```python
from build123d import *

# Parameters (mm, degrees)
SKETCH1_R                = 14.2875
BOSS_EXTRUDE2_DEPTH      = 3.175
BOSS_EXTRUDE2_DEPTH_BACK = 3.175


with BuildPart() as part:
    # Sketch1 → Boss-Extrude2 (new body, two sides)
    with BuildSketch(Plane(origin=(0, 0, 0), x_dir=(0, 0, -1), z_dir=(1, 0, 0))) as boss_extrude2_sk:
        with BuildLine():
            Line((10.594785966, 15.13092246), (203.963780766, 291.290466949))
            Line((203.963780766, 291.290466949), (110.334702104, 356.850253624))
            Line((110.334702104, 356.850253624), (-84.6362425, 78.402887714))
            ThreePointArc((-84.6362425, 78.402887714), (-88.561708566, 58.046841565), (-76.011825816, 41.54598275))
            Line((-76.011825816, 41.54598275), (-16.208376106, 8.859054586))
            ThreePointArc((-16.208376106, 8.859054586), (-1.608360556, 6.873414672), (10.594785966, 15.13092246))
        make_face()
        with Locations((-62.285836902, 68.806748098)):
            Circle(SKETCH1_R, mode=Mode.SUBTRACT)
        with Locations((-5.068066609, 28.742434019)):
            Circle(SKETCH1_R, mode=Mode.SUBTRACT)
        with Locations((-29.716861807, 107.792666854)):
            Circle(SKETCH1_R, mode=Mode.SUBTRACT)
    extrude(amount=BOSS_EXTRUDE2_DEPTH)
    extrude(boss_extrude2_sk.sketch, amount=-BOSS_EXTRUDE2_DEPTH_BACK)


solid = part.part
```
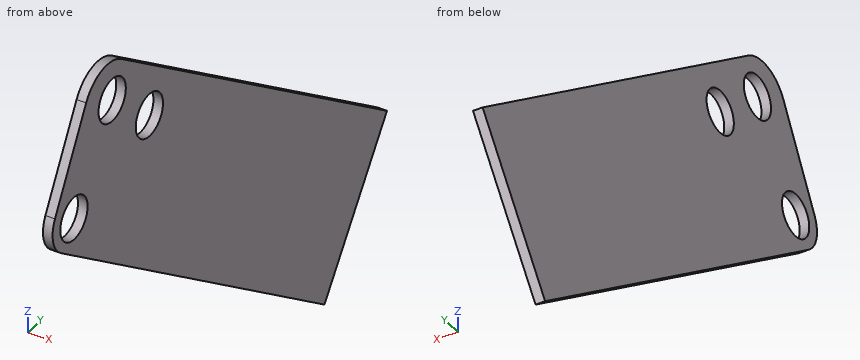
Geometry: final body of the model. Coordinates: model frame, mm. Round coordinates to 2 decimals unless told otherwise and drop trailing zeros. Write each loop counter-clockwise with the first axis right and the second up, starting at its lowest first coordinate (ties: lowest second). Pieces come first, ordered by that corner, then holes. Notation, with made-up numbers: (-1, 34) -> (22, 34) arc R31 cw to (22, 61) -> close; hole circle Ø11 at (47, 54.5). An arc over 180 degrees is marked (long way). Return JSON: item names as keys, results as strings.
Q1. First-contact query: pin 1 Ø3 at (x, z) = (0.5, 49) entering from -Y; pin 2 Ø1 at (x, y) = (0, 127) entering from -Z; pin 3 Ø2 at (x, z) = (2, -153.5) entering from +Y. Flat tips, straight axial feed; report the tip coordinate or a pass-through.
From the geometry:
{"pin 1": "y = 25.96", "pin 2": "z = -89.28", "pin 3": "y = 327.33"}
Q2. Section A-A on y = 102.5. Return the cut outline in (x, z) (3 decimals), and give its area (3 significant figures).
From the geometry:
{"outline": "(-3.175, -71.771) -> (3.175, -71.771) -> (3.175, 16.446) -> (-3.175, 16.446) -> close; (-3.175, 42.988) -> (3.175, 42.988) -> (3.175, 67.763) -> (-3.175, 67.763) -> close", "area": "718 mm2"}
Q3. Section B-B on z = 55. Return the cut outline in (x, y) (1 decimal), and give its area (3 significant figures).
From the geometry:
{"outline": "(-3.2, 30.1) -> (3.2, 30.1) -> (3.2, 56.5) -> (-3.2, 56.5) -> close; (-3.2, 81.1) -> (3.2, 81.1) -> (3.2, 120.7) -> (-3.2, 120.7) -> close", "area": "420 mm2"}
Q4. Section C-C on x = -0.5. Return the cut outline in (y, z) (1 decimal).
From the geometry:
{"outline": "(8.9, 16.2) arc R20.6 ccw to (15.1, -10.6) -> (291.3, -204) -> (356.9, -110.3) -> (78.4, 84.6) arc R25.4 ccw to (41.5, 76) -> close; hole circle Ø28.6 at (28.7, 5.1); hole circle Ø28.6 at (68.8, 62.3); hole circle Ø28.6 at (107.8, 29.7)"}
Q5. Ray query, line 1 (Z direction, x = 0, y = 37); line 2 (Z direction, x = 0, y = 61.5); line 3 (Y direction, x = -2.25, z = 32). Return the intervals inside material, ascending.
From the geometry:
{"line 1": "-25.91 to -6.59, 16.73 to 67.69", "line 2": "-43.06 to 50.01, 74.56 to 89.12", "line 3": "17.49 to 93.69, 121.9 to 153.58"}
Q6. Section D-D on z = -122. Return the cut outline in (x, y) (3 decimals), and give its area (3 significant figures).
From the geometry:
{"outline": "(-3.175, 174.234) -> (3.175, 174.234) -> (3.175, 348.682) -> (-3.175, 348.682) -> close", "area": "1,110 mm2"}
